```python
from build123d import *

# Parameters (mm, degrees)
ESQUISSE1_W                = 75
ESQUISSE1_H                = 63
BOSS_EXTRU_1_DEPTH         = 1100
R_P_TITION_LIN_AIRE2_COUNT = 2
R_P_TITION_LIN_AIRE2_PITCH = 375
ESQUISSE3_W                = 75
ESQUISSE3_H                = 63
BOSS_EXTRU_2_DEPTH         = 512.5
BOSS_EXTRU_3_DEPTH         = 182.5
BOSS_EXTRU_3_DEPTH_BACK    = 192.5
ESQUISSE4_W                = 75
ESQUISSE4_H                = 63
ESQUISSE5_W                = 75
ESQUISSE5_H                = 63
BOSS_EXTRU_4_DEPTH         = 500


with BuildPart() as part:
    # Esquisse1 → Boss.-Extru.1 (new body)
    with BuildSketch(Plane.XY):
        with Locations((37.5, 31.5)):
            Rectangle(ESQUISSE1_W, ESQUISSE1_H)
    extrude(amount=BOSS_EXTRU_1_DEPTH)


with BuildPart() as r_p_tition_lin_aire2_1:
    # R_p_tition lin_aire2: pattern copy
    add(part.part.moved(Location(Vector(-1, 0, 0) * (1 * R_P_TITION_LIN_AIRE2_PITCH))))


with BuildPart() as body_3:
    # Esquisse3 → Boss.-Extru.2 (new body)
    with BuildSketch(Plane.XY):
        with Locations((-155, 31.5)):
            Rectangle(ESQUISSE3_W, ESQUISSE3_H)
    extrude(amount=BOSS_EXTRU_2_DEPTH)


with BuildPart() as part_1:
    add(part.part)

    add(r_p_tition_lin_aire2_1.part)  # Boss.-Extru.3 merges R_p_tition lin_aire2_1

    add(body_3.part)  # Boss.-Extru.3 merges body 3
    # Esquisse4 → Boss.-Extru.3 (add, two sides: drawn at the far end of the back side and taken through both)
    with BuildSketch(Plane.ZY.offset(192.5).offset(-BOSS_EXTRU_3_DEPTH_BACK)):
        with Locations((550, 31.5)):
            Rectangle(ESQUISSE4_W, ESQUISSE4_H)
    extrude(amount=BOSS_EXTRU_3_DEPTH + BOSS_EXTRU_3_DEPTH_BACK)

    # Esquisse5 → Boss.-Extru.4 (add)
    with BuildSketch(Plane.ZY.offset(375)):
        with Locations((-37.5, 31.5)):
            Rectangle(ESQUISSE5_W, ESQUISSE5_H)
    extrude(amount=-BOSS_EXTRU_4_DEPTH)


solid = part_1.part
```
Input: part model. Units: mm. Frame: model coordinates. A direction names the side the tool comes from. Round coordinates to 2 decimals unless told otherwise and drop trailing zeros. Loops run counter-clockwise (first coordinate to the right, second up) from the corner with the lowest first, then second, coordinate; pieces in that order, holes last. Notation, with made-up numbers: M 25.5,69 L 30.5,69 A17 cw 30.5,95 Z; hole C 26,37 d11. An arc over 180 degrees is marked long. Answer in a Markdown table with one row per item. Add a question column.
1. Ray query, probe 1 along X at (y, z) = (49, 265); probe 2 along Z at (x, y) = (-296, 26); probe 3 along X at (y, z) = (10.5, 1026). Return the intervals inside material, ascending.
2. Section A-A (x = -44). Output: boundary loops of the cut face in (y, z).
3. Contact query for flat-ended pins moving along their axis: pin 1 (3 mm diameter, centred on x = -223, y = 14, fed in from +Z); pin 2 (19 mm diameter, centred on y = 24.5, z = 268.5, fed in from +X). Output: stop coordinate, or through.
4. Section B-B (z = 247). Output: boundary loops of the cut face in (x, y), and give its area (3 significant figures).
5. Section D-D (z = 848). Output: boundary loops of the cut face in (x, y).
6. Set-up query: faces 5 (the face through (-60, 31, 0)), 6 (the face through (-148, 31, 587.5)), 7 (the face through (100, 31, 0)). Return all of +Z, -Z, +X, -X, +Y, -Y with unobstructed straight access to the full face (end or side cutting, diameter ignored); none if empty.
7. Section C-C (y = 52). Output: boundary loops of the cut face in (x, z).
8. Mould query, pull axis X, two halves, no side actions, for faces 1 (the face through (0, 31, 840)), 2 (the face through (-375, 32, 504)), 3 (the face through (-300, 31, 840)), 4 (the face through (37, 32, 1100)). Classes: released by +X, released by -X, zero draft, split by the parting line, or undercut.
Values follow:
| question | item | result |
|---|---|---|
| 1 | probe 1 | -375 to -300, -192.5 to -117.5, 0 to 75 |
| 1 | probe 2 | -75 to 0, 512.5 to 587.5 |
| 1 | probe 3 | -375 to -300, 0 to 75 |
| 2 | outline | M 0,-75 L 63,-75 L 63,0 L 0,0 Z; M 0,512.5 L 63,512.5 L 63,587.5 L 0,587.5 Z |
| 3 | pin 1 | z = 587.5 |
| 3 | pin 2 | x = 75 |
| 4 | outline | M -375,0 L -300,0 L -300,63 L -375,63 Z; M -192.5,0 L -117.5,0 L -117.5,63 L -192.5,63 Z; M 0,0 L 75,0 L 75,63 L 0,63 Z |
| 4 | area | 14,200 mm^2 |
| 5 | outline | M -375,0 L -300,0 L -300,63 L -375,63 Z; M 0,0 L 75,0 L 75,63 L 0,63 Z |
| 6 | face 5 | +Y, -Y |
| 6 | face 6 | +Z, +Y, -Y |
| 6 | face 7 | +Z, +X, +Y, -Y |
| 7 | outline | M -375,-75 L 125,-75 L 125,0 L 75,0 L 75,1100 L 0,1100 L 0,587.5 L -300,587.5 L -300,1100 L -375,1100 Z; hole M -300,0 L -192.5,0 L -192.5,512.5 L -300,512.5 Z; hole M -117.5,0 L 0,0 L 0,512.5 L -117.5,512.5 Z |
| 8 | face 1 | undercut |
| 8 | face 2 | released by -X |
| 8 | face 3 | undercut |
| 8 | face 4 | zero draft |
